from build123d import *

# Parameters (mm, degrees)
SKETCH_R  = 2.15
PAD_DEPTH = 2


with BuildPart() as part:
    # Sketch → Pad (new body)
    with BuildSketch(Plane.XY):
        with BuildLine():
            ThreePointArc((0, 5), (-3.043807, 3.966767), (-4.829629, 1.294095))
            Line((-13.111839, -29.615531), (-4.829629, 1.294095))
            ThreePointArc((-13.111839, -29.615531), (-11.610103, -34.641265), (-6.445927, -35.560225))
            Line((71.836283, -4.650598), (-6.445927, -35.560225))
            ThreePointArc((71.836283, -4.650598), (74.911873, 0.934614), (70, 5))
            Line((0, 5), (70, 5))
        make_face()
        Circle(SKETCH_R, mode=Mode.SUBTRACT)
        with Locations((-8.282209, -30.909626)):
            Circle(SKETCH_R, mode=Mode.SUBTRACT)
        with Locations((70, 0)):
            Circle(SKETCH_R, mode=Mode.SUBTRACT)
        with BuildLine():
            Line((2.1675, -23.558181), (54.587435, -2.860239))
            ThreePointArc((54.587435, -2.860239), (55.817671, -0.626154), (53.852922, 1))
            Line((53.852922, 1), (8.513638, 1))
            ThreePointArc((8.513638, 1), (6.078592, 0.173413), (4.649935, -1.964724))
            Line((4.649935, -1.964724), (-0.498864, -21.180304))
            ThreePointArc((-0.498864, -21.180304), (0.10183, -23.190597), (2.1675, -23.558181))
        make_face(mode=Mode.SUBTRACT)
    extrude(amount=PAD_DEPTH)


solid = part.part
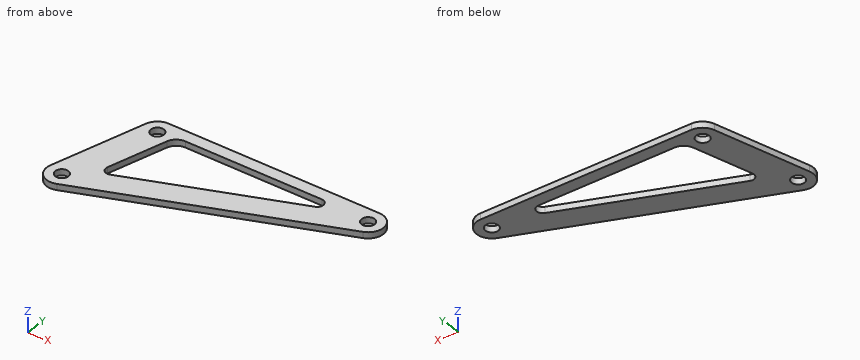
Could you check a few things on this model? Use its own coordinates, in mm. Give positions to 0.01 mm unless a question says otherwise; leave off trailing zeros. Write each loop counter-clockwise with the first axis right and the second up, starting at its lowest first coordinate (ties: lowest second). Pieces come first, ordered by that corner, then holes. Notation, with made-up numbers: (55, 9) -> (71, 9) arc R24 ccw to (71, 34) -> close; hole circle Ø1 at (-7.5, 16.5). An arc over 180 degrees is marked (long way). Answer as CSV lines item,"result". Start each with the question number.
(1) If we section it at B-B, the plane y = 0: Write out the boundary of the cut face in (x, z).
(2) If we section it at C-C, the plane z = 1.6: Write out the boundary of the cut face in (x, y).
(3) If we section it at A-A, the plane x = 43: Write out the boundary of the cut face in (y, z).
(4) If we section it at D-D, the plane y = -18.5: Write out the boundary of the cut face in (x, z), and give its area (3 significant figures).
(5) I'm going to push flat-ended pins straight in: pin 1 Ø1 at (x, y) = (58, -2) entering from -Z; pin 2 Ø0.6 at (x, z) = (37, 0.5) entering from -Y. Where does each tip first touch, or does it pass through?
(6) Please list where these lines run through material, in increasing order: line 1 (X direction, y = -1, z = 1.5); line 2 (Y direction, x = 6, z = 0.8); line 3 (Y direction, x = 37.5, z = 1.2).
Answer list:
1,outline,"(-5.18, 0) -> (-2.15, 0) -> (-2.15, 2) -> (-5.18, 2) -> close; (2.15, 0) -> (5.87, 0) -> (5.87, 2) -> (2.15, 2) -> close; (55.58, 0) -> (67.85, 0) -> (67.85, 2) -> (55.58, 2) -> close; (72.15, 0) -> (75, 0) -> (75, 2) -> (72.15, 2) -> close"
2,outline,"(-13.11, -29.62) arc R5 ccw to (-6.45, -35.56) -> (71.84, -4.65) arc R5 ccw to (70, 5) -> (0, 5) arc R5 ccw to (-4.83, 1.29) -> close; hole circle Ø4.3 at (-8.28, -30.91); hole circle Ø4.3 at (0, 0); hole (-0.5, -21.18) arc R2 ccw to (2.17, -23.56) -> (54.59, -2.86) arc R2 ccw to (53.85, 1) -> (8.51, 1) arc R4 ccw to (4.65, -1.96) -> close; hole circle Ø4.3 at (70, 0)"
3,outline,"(-16.04, 0) -> (-7.44, 0) -> (-7.44, 2) -> (-16.04, 2) -> close; (1, 0) -> (5, 0) -> (5, 2) -> (1, 2) -> close"
4,outline,"(-10.13, 0) -> (0.22, 0) -> (0.22, 2) -> (-10.13, 2) -> close; (14.98, 0) -> (36.76, 0) -> (36.76, 2) -> (14.98, 2) -> close"
4,area,"64.3 mm^2"
5,pin 1,"z = 0"
5,pin 2,"y = -18.52"
6,line 1,"-5.44 to -1.9, 1.9 to 5.05, 55.85 to 68.1, 71.9 to 74.9"
6,line 2,"-30.65 to -22.04, 0.11 to 5"
6,line 3,"-18.21 to -9.61, 1 to 5"
